from build123d import *

# Parameters (mm, degrees)
SKETCH_1_R      = 71
SKETCH_1_R_2    = 63.5
EXTRUDE_1_DEPTH = 3
SKETCH_2_R      = 71
SKETCH_2_R_2    = 68
EXTRUDE_2_DEPTH = 8
EXTRUDE_START   = -11
SKETCH_3_R      = 1.25
EXTRUDE_3_DEPTH = 11
FILLET_2_R      = 3


with BuildPart() as part:
    # 草图1 → 凸台-拉伸1 (new body)
    with BuildSketch(Plane.XY):
        Circle(SKETCH_1_R)
        Circle(SKETCH_1_R_2, mode=Mode.SUBTRACT)
    extrude(amount=EXTRUDE_1_DEPTH)

    # 草图2 → 凸台-拉伸2 (add)
    with BuildSketch(Plane.XY.offset(3)):
        Circle(SKETCH_2_R)
        Circle(SKETCH_2_R_2, mode=Mode.SUBTRACT)
    extrude(amount=EXTRUDE_2_DEPTH)

    # 草图3 → 凸台-拉伸3 (add)
    # profile 1 of 6: a face of its own
    with BuildSketch(Plane.XY.offset(11).offset(EXTRUDE_START)):
        with BuildLine():
            ThreePointArc((2.5, 74), (0, 76.5), (-2.5, 74))
            Line((-2.5, 74), (-2.5, 70.955972264))
            ThreePointArc((-2.5, 70.955972264), (-0.051390082, 70.999981402), (2.397280978, 70.959516937))
            Line((2.397280978, 70.959516937), (2.5, 74))
        make_face()
        with Locations((0, 74)):
            Circle(SKETCH_3_R, mode=Mode.SUBTRACT)
    # profile 2 of 6: a face of its own
    with BuildSketch(Plane.XY.offset(11).offset(EXTRUDE_START)):
        with BuildLine():
            ThreePointArc((65.33587988, 34.834936491), (66.25094339, 38.25), (62.83587988, 39.165063509))
            Line((62.83587988, 39.165063509), (60.199674531, 37.643049642))
            ThreePointArc((60.199674531, 37.643049642), (61.462092521, 35.544495818), (62.651384796, 33.403652242))
            Line((62.651384796, 33.403652242), (65.33587988, 34.834936491))
        make_face()
        with Locations((64.08587988, 37)):
            Circle(SKETCH_3_R, mode=Mode.SUBTRACT)
    # profile 3 of 6: a face of its own
    with BuildSketch(Plane.XY.offset(11).offset(EXTRUDE_START)):
        with BuildLine():
            ThreePointArc((62.83587988, -39.165063509), (66.25094339, -38.25), (65.33587988, -34.834936491))
            Line((65.33587988, -34.834936491), (62.699674531, -33.312922623))
            ThreePointArc((62.699674531, -33.312922623), (61.513482603, -35.455485584), (60.254103819, -37.555864695))
            Line((60.254103819, -37.555864695), (62.83587988, -39.165063509))
        make_face()
        with Locations((64.08587988, -37)):
            Circle(SKETCH_3_R, mode=Mode.SUBTRACT)
    # profile 4 of 6: a face of its own
    with BuildSketch(Plane.XY.offset(11).offset(EXTRUDE_START)):
        with BuildLine():
            ThreePointArc((-2.5, -74), (0, -76.5), (2.5, -74))
            Line((2.5, -74), (2.5, -70.955972264))
            ThreePointArc((2.5, -70.955972264), (0.051390082, -70.999981402), (-2.397280978, -70.959516937))
            Line((-2.397280978, -70.959516937), (-2.5, -74))
        make_face()
        with Locations((0, -74)):
            Circle(SKETCH_3_R, mode=Mode.SUBTRACT)
    # profile 5 of 6: a face of its own
    with BuildSketch(Plane.XY.offset(11).offset(EXTRUDE_START)):
        with BuildLine():
            ThreePointArc((-65.33587988, -34.834936491), (-66.25094339, -38.25), (-62.83587988, -39.165063509))
            Line((-62.83587988, -39.165063509), (-60.199674531, -37.643049642))
            ThreePointArc((-60.199674531, -37.643049642), (-61.462092521, -35.544495818), (-62.651384796, -33.403652242))
            Line((-62.651384796, -33.403652242), (-65.33587988, -34.834936491))
        make_face()
        with Locations((-64.08587988, -37)):
            Circle(SKETCH_3_R, mode=Mode.SUBTRACT)
    # profile 6 of 6: a face of its own
    with BuildSketch(Plane.XY.offset(11).offset(EXTRUDE_START)):
        with BuildLine():
            ThreePointArc((-62.83587988, 39.165063509), (-66.25094339, 38.25), (-65.33587988, 34.834936491))
            Line((-65.33587988, 34.834936491), (-62.699674531, 33.312922623))
            ThreePointArc((-62.699674531, 33.312922623), (-61.513482603, 35.455485584), (-60.254103819, 37.555864695))
            Line((-60.254103819, 37.555864695), (-62.83587988, 39.165063509))
        make_face()
        with Locations((-64.08587988, 37)):
            Circle(SKETCH_3_R, mode=Mode.SUBTRACT)
    extrude(amount=EXTRUDE_3_DEPTH)

    # 圆角2
    fillet_2_edges = [part.edges().sort_by_distance(p)[0] for p in [
        (60.254103819, -37.555864695, 5.5),
        (62.699674531, -33.312922623, 5.5),
        (-2.397280978, -70.959516937, 5.5),
        (2.5, -70.955972264, 5.5),
        (-62.651384796, -33.403652242, 5.5),
        (-60.199674531, -37.643049642, 5.5),
        (-60.254103819, 37.555864695, 5.5),
        (-62.699674531, 33.312922623, 5.5),
        (2.397280978, 70.959516937, 5.5),
        (-2.5, 70.955972264, 5.5),
        (62.651384796, 33.403652242, 5.5),
        (60.199674531, 37.643049642, 5.5),
    ]]
    fillet(fillet_2_edges, radius=FILLET_2_R)


solid = part.part
For this review, take the finished solid that the model builds, in its own axes (mm). Round coordinates to 2 decimals unless told otherwise and drop trailing zeros. Loops run counter-clockwise (first coordinate to the right, second up) from the corner with the lowest first, then second, coordinate; pieces in that order, holes last. Notation, with made-up numbers: (50.25, 25.25) - (103.25, 25.25) arc R26 ccw to (103.25, 60.25) - close; hole circle Ø5 at (58, 2.25). An arc over 180 degrees is marked (long way). Use one line per item in the form item = value.
1) Mouldability with a two-part tool opening along Y and no side actions: class faces 1 (the face through (35.11, -61.71, 5.42)), 2 (the face through (66.28, 38.2, 5.42)), 3 (the face through (66.22, -38.3, 5.42)), 4 (the face through (-16, -62, 0)) as pulls with the +Y half, pulls with the -Y half, needs draft (parallel to the pull), parting line crosses it, or undercut.
Solutions:
face_1 = pulls with the -Y half
face_2 = undercut
face_3 = undercut
face_4 = needs draft
2) Wall thickness on probe 1 along X at (y, z) = (0.5, 4.5); probe 2 along X at (y, z) = (-74, 6.5); probe 3 along Y at (x, z) = (-48.5, 8.5): over which ranges is each line inside the solid? List them lowest first.
Solutions:
probe_1 = -71 to -68, 68 to 71
probe_2 = -2.5 to -1.25, 1.25 to 2.5
probe_3 = -51.85 to -47.66, 47.66 to 51.85
3) We need section A-A on y = 52. Write out the cut boundary in (x, z).
Solutions:
outline = (-48.34, 0) - (-36.45, 0) - (-36.45, 3) - (-43.82, 3) - (-43.82, 11) - (-48.34, 11) - close; (36.45, 0) - (48.34, 0) - (48.34, 11) - (43.82, 11) - (43.82, 3) - (36.45, 3) - close
4) Clearance check with flat-ended pins moving along their axes: P1, Ø6, axis at y = -22, z = 2.5, coming from the -X side; P2, Ø1.5, axis at y = -54.5, z = 8.5, coming from the -X side; P3, Ø5, axis at y = -14.5, z = 9.5, coming from the +X side; P4, Ø2, axis at x = -64.09, y = -37, coming from the +Z side (3 decimals). State where each tip first meets the part, or that it passes through.
Solutions:
P1 = -68.41
P2 = -46.39
P3 = 69.98
P4 = through
5) We need section C-C on z = 6.5. State how many separate pieces and enclosed holes the cut face has, then the cut area to 3 significant figures.
Solutions:
separate_pieces = 1
enclosed_holes = 7
area = 1,450 mm2
6) We need section B-B on x = -19.5. Write out the cut boundary in (y, z), then the cut area to 3 significant figures.
Solutions:
outline = (-68.27, 0) - (-60.43, 0) - (-60.43, 3) - (-65.14, 3) - (-65.14, 11) - (-68.27, 11) - close; (60.43, 0) - (68.27, 0) - (68.27, 11) - (65.14, 11) - (65.14, 3) - (60.43, 3) - close
area = 97.0 mm2
